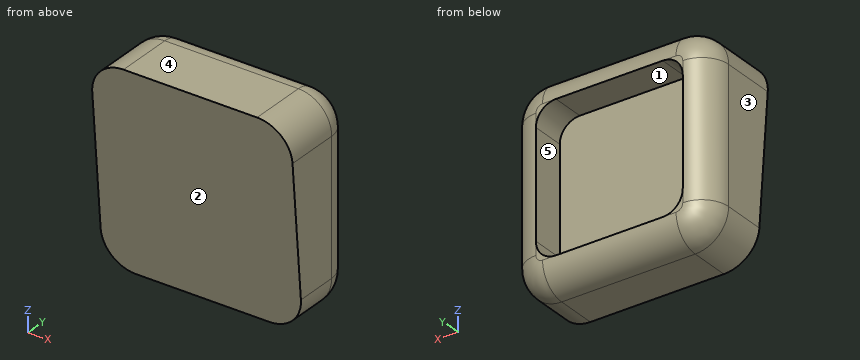
from build123d import *

# Parameters (mm, degrees)
SKETCH1_W           = 30
SKETCH1_H           = 10
BOSS_EXTRUDE1_DEPTH = 30
SKETCH2_W           = 22
SKETCH2_H           = 22
CUT_EXTRUDE1_DEPTH  = 5
FILLET1_R           = 5
FILLET2_R           = 3
FILLET3_R           = 4


with BuildPart() as part:
    # Sketch1 → Boss-Extrude1 (new body)
    with BuildSketch(Plane(origin=(0, 0, 0), x_dir=(0, 0, -1), z_dir=(1, 0, 0))):
        Polygon((-15, -5), (-15, -7.625), (15, -5), align=None)
        Rectangle(SKETCH1_W, SKETCH1_H)
    extrude(amount=BOSS_EXTRUDE1_DEPTH)

    # Sketch2 → Cut-Extrude1 (cut)
    with BuildSketch(Plane(origin=(0, 5, 0), x_dir=(1, 0, 0), z_dir=(0, 1, 0))):
        with Locations((15, 0)):
            Rectangle(SKETCH2_W, SKETCH2_H)
    extrude(amount=-CUT_EXTRUDE1_DEPTH, mode=Mode.SUBTRACT)

    # Fillet1
    fillet1_edges = [part.edges().sort_by_distance(p)[0] for p in [
        (30, 0, -15),
        (30, -1.3125, 15),
        (0, 0, -15),
        (0, -1.3125, 15),
    ]]
    fillet(fillet1_edges, radius=FILLET1_R)

    # Fillet2
    fillet2_edges = [part.edges().sort_by_distance(p)[0] for p in [
        (26, 2.5, 11),
        (4, 2.5, 11),
        (4, 2.5, -11),
        (26, 2.5, -11),
    ]]
    fillet(fillet2_edges, radius=FILLET2_R)

    # Fillet3
    fillet3_edges = [part.edges().sort_by_distance(p)[0] for p in [
        (15, 5, 15),
        (0, 5, 0),
        (30, 5, 0),
        (15, 5, -15),
        (28.535533906, 5, 13.535533906),
        (28.535533906, 5, -13.535533906),
        (1.464466094, 5, -13.535533906),
        (1.464466094, 5, 13.535533906),
    ]]
    fillet(fillet3_edges, radius=FILLET3_R - 0.0001)  # a hair under: the kernel refuses the full size


solid = part.part
CAD build for the part. Positions are in the model's coordinates, mm. Face numbers are marked on the shaded views. A direction names the side the tool comes from. Round coordinates to 2 decimals unless told otherwise and drop trailing zeros. Loops run counter-clockwise (first coordinate to the right, second up) from the corner with the lowest first, then second, coordinate; pieces in that order, holes last.
(1) Two-plate mould, pull along X, no slides. Class the marked faces 3, 4 and 5: +X half, -X half, draft (parallel to the pull), parting line (faces both ways), or undercut.
(2) Which spindle directions (+Z, -Z, +X, -X, +Y, -Y) get a long thin tool onto all of the face, cutting with end or side? Do the marked faces 1 and 2. Say none if no direction does.
(3) Cut at C-C (x = 24). Give the cut face in (y, z) (3 decimals).
(4) Wall check: line 1 along Z through (x, y) = (21, 0.75); line 2 along X through (y, z) = (0.5, 5.75); line 3 along X through (y, z) = (3.5, 8.75). Give the ranges that are in metal, low to high.
(5) Drop flat-ended pins along their axis: pin 1 (3 mm diameter, centred on x = 10, z = 9, fed in from -Y); pin 2 (2.5 mm diameter, centred on y = 3, z = 3, fed in from -X); pin 3 (6.5 mm diameter, centred on x = 15, z = 1.5, fed in from +Y). Give the stop position or say it passes through.
(6) Cut at A-A (y = -3). Give the cut face in (x, z), plus the area to 3 significant figures.
Findings below:
1. face 3: -X half
1. face 4: draft
1. face 5: undercut
2. face 1: +Y
2. face 2: -Z, +X, -X, -Y
3. outline: (-7.625, 15) - (-5, -15) - (1, -15) arc R4 ccw to (5, -11) - (5, -10.828) - (0, -10.828) - (0, 10.828) - (5, 10.828) - (5, 11) arc R4 ccw to (1, 15) - close
4. line 1: z = -15 to -11, 11 to 15
4. line 2: x = 0 to 4, 26 to 30
4. line 3: x = 0.88 to 4.1, 25.9 to 29.12
5. pin 1: stops at y = -7.23
5. pin 2: stops at x = 0.07
5. pin 3: stops at y = 0
6. outline: (0, -10) arc R5 ccw to (5, -15) - (25, -15) arc R5 ccw to (30, -10) - (30, 10) arc R5 ccw to (25, 15) - (5, 15) arc R5 ccw to (0, 10) - close
6. area: 879 mm2
